Check sheet for the modelled part. Datum: model origin and axes. Units: mm. A direction names the side the tool comes from. Coordinates: 2 decimals unless noted, no trailing zeros. Order: outer loops, then holes, each group sorted by start corner. A loop starts at its lowest first (then second) coordinate and runs counter-clockwise, first axis right, second up.
from build123d import *

# Parameters (mm, degrees)
SKETCH_1_W      = 160
SKETCH_1_H      = 80
EXTRUDE_1_DEPTH = 10
SKETCH_2_R      = 8
EXTRUDE_2_DEPTH = 150
SKETCH_3_R      = 7.5
EXTRUDE_3_DEPTH = 15
EXTRUDE_START   = -15
SKETCH_4_R      = 7.5
EXTRUDE_4_DEPTH = 15


with BuildPart() as part:
    # 草图1 → 凸台-拉伸1 (new body)
    with BuildSketch(Plane(origin=(0, 0, 0), x_dir=(1, 0, 0), z_dir=(0, 1, 0))):
        Rectangle(SKETCH_1_W, SKETCH_1_H)
    extrude(amount=EXTRUDE_1_DEPTH)

    # 草图2 → 凸台-拉伸2 (add)
    with BuildSketch(Plane.XZ):
        with Locations(Location((0, 25, 0), (0, 0, 90))):
            Circle(SKETCH_2_R)
        with Locations(Location((0, -25, 0), (0, 0, 90))):
            Circle(SKETCH_2_R)
    extrude(amount=EXTRUDE_2_DEPTH)

    # 草图3 → 凸台-拉伸3 (add)
    with BuildSketch(Plane(origin=(0, 0, -40), x_dir=(-1, 0, 0), z_dir=(0, 0, -1))):
        with Locations((0, -142.5)):
            Circle(SKETCH_3_R)
    extrude(amount=-EXTRUDE_3_DEPTH)

    # 草图4 → 凸台-拉伸4 (add)
    with BuildSketch(Plane.XY.offset(40).offset(EXTRUDE_START)):
        with Locations(Location((0, -142.5, 0), (0, 0, 180))):
            Circle(SKETCH_4_R)
    extrude(amount=EXTRUDE_4_DEPTH)


solid = part.part
(1) Cross-section at B-B (z = -25). Enter the section's corners in (x, y).
Filled in:
outline: (-80, 0) - (-8, 0) - (-8, -150) - (8, -150) - (8, 0) - (80, 0) - (80, 10) - (-80, 10) - close
(2) Thickness scan on probe 1 along Y at (x, z) = (56.5, -10); probe 2 along Y at (x, z) = (-3, 33); probe 3 along X at (y, z) = (-107, 20) (3 decimals). Record the ranges inside material, lowest first.
Filled in:
probe 1: y = 0 to 10
probe 2: y = -149.37 to -135.63, 0 to 10
probe 3: x = -6.245 to 6.245
(3) Release check for a two-part mould opening along Y. For faces 1 (the cylindrical face through (0, -74, 17)), 2 (the flat face through (0, -150, -25)), 3 (the flat face through (0, -143, 40)) record: +Y half, -Y half, draft (parallel to the pull), parting line (faces both ways), or undercut.
Filled in:
face 1: undercut
face 2: -Y half
face 3: draft
(4) Cross-section at D-D (y = -124.5). Enter the section's corners in (x, z).
Filled in:
outline: circle Ø16 at (0, -25); circle Ø16 at (0, 25)
(5) Go/stop test with flat-tipped pins: P1, Ø5, axis at x = 39.5, z = 17.5, coming from the -Y side; P2, Ø4, axis at y = -105.5, z = 31, coming from the +X side; P3, Ø5, axis at x = 7.5, y = -95.5, coming from the -Z side (3 decimals). Record where each tip stops, or that it passes through.
Filled in:
P1: stops at y = 0
P2: stops at x = 6.93
P3: stops at z = -31.245
(6) Tool access check on faces 4 (the cylindrical face through (3.06, -73.95, -17.61)), 5 (the cylindrical face through (7.493, -142.17, -35.335)), 6 (the cylindrical face through (7.493, -142.83, 35.164)). Record the directions out of +Z, -Z, +X, -X, +Y, -Y that give a thin tool (end or side, any length) a straight path to the whole face; none if there is none.
Filled in:
face 4: none
face 5: -Z
face 6: +Z
(7) Cross-section at C-C (x = -68). Enter the section's corners in (y, z).
Filled in:
outline: (0, -40) - (10, -40) - (10, 40) - (0, 40) - close
(8) Cross-section at A-A (y = -142.5). Enter the section's corners in (x, z), and give its area (3 significant figures).
Filled in:
outline: (-7.5, -40) - (7.5, -40) - (7.5, -27.78) arc R8 ccw (long way) to (-7.5, -27.78) - close; (-7.5, 27.78) arc R8 ccw (long way) to (7.5, 27.78) - (7.5, 40) - (-7.5, 40) - close
area: 655 mm2
